```python
from build123d import *

# Parameters (mm, degrees)
F0_R     = 1.397
F1_DEPTH = 3.048


with BuildPart() as f1:
    # F0 (on Front) → F1 (new body)
    with BuildSketch(Plane.XZ):
        with BuildLine():
            ThreePointArc((3.175, 66.675), (-2.245064, 68.920064), (0, 63.5))
            ThreePointArc((0, 63.5), (2.245064, 64.429936), (3.175, 66.675))
        make_face()
        with BuildLine():
            ThreePointArc((0, 57.15), (6.735192, 59.939808), (9.525, 66.675))
            ThreePointArc((9.525, 66.675), (0.596483, 76.181305), (-9.450293, 67.865625))
            ThreePointArc((-9.450293, 67.865625), (-7.14375, 60.374805), (0, 57.15))
        make_face()
        with BuildLine():
            ThreePointArc((3.175, 66.675), (2.245064, 64.429936), (0, 63.5))
            ThreePointArc((0, 63.5), (-2.245064, 68.920064), (3.175, 66.675))
        make_face(mode=Mode.SUBTRACT)
        with BuildLine():
            Line((15.747457, 17.883289), (9.525, 66.675))
            ThreePointArc((9.525, 66.675), (6.735192, 59.939808), (0, 57.15))
            Line((0, 57.15), (0, 31.75))
            ThreePointArc((0, 31.75), (10.491283, 27.789219), (15.747457, 17.883289))
        make_face()
        with BuildLine():
            ThreePointArc((0, 57.15), (-7.14375, 60.374805), (-9.450293, 67.865625))
            Line((-9.450293, 67.865625), (-15.750488, 17.859375))
            ThreePointArc((-15.750488, 17.859375), (-10.500326, 27.78125), (0, 31.75))
            Line((0, 31.75), (0, 57.15))
        make_face()
        with Locations((-3.175, 52.4002)):
            Circle(F0_R, mode=Mode.SUBTRACT)
        with BuildLine():
            ThreePointArc((15.875, 15.875), (15.843082, 16.881168), (15.747457, 17.883289))
            ThreePointArc((15.747457, 17.883289), (10.491283, 27.789219), (0, 31.75))
            Line((0, 31.75), (0, 17.653))
            ThreePointArc((0, 17.653), (1.257236, 17.132236), (1.778, 15.875))
            ThreePointArc((1.778, 15.875), (1.257236, 14.617764), (0, 14.097))
            Line((0, 14.097), (0, 0))
            ThreePointArc((0, 0), (10.572083, 4.03242), (15.77332, 14.081125))
            ThreePointArc((15.77332, 14.081125), (15.84956, 14.976623), (15.875, 15.875))
        make_face()
        with BuildLine():
            ThreePointArc((0, 31.75), (-10.500326, 27.78125), (-15.750488, 17.859375))
            ThreePointArc((-15.750488, 17.859375), (-15.875, 15.875), (-15.750488, 13.890625))
            ThreePointArc((-15.750488, 13.890625), (-10.500326, 3.96875), (0, 0))
            Line((0, 0), (0, 14.097))
            ThreePointArc((0, 14.097), (-1.778, 15.875), (0, 17.653))
            Line((0, 17.653), (0, 31.75))
        make_face()
        with BuildLine():
            ThreePointArc((0, 0), (-10.500326, 3.96875), (-15.750488, 13.890625))
            Line((-15.750488, 13.890625), (-8.643798, -48.607884))
            ThreePointArc((-8.643798, -48.607884), (-6.48968, -41.831439), (0, -38.9255))
            Line((0, -38.9255), (0, 0))
        make_face()
        with BuildLine():
            Line((10.715191, -30.394381), (15.77332, 14.081125))
            ThreePointArc((15.77332, 14.081125), (10.572083, 4.03242), (0, 0))
            Line((0, 0), (0, -38.9255))
            ThreePointArc((0, -38.9255), (0.148885, -38.926774), (0.297726, -38.930596))
            ThreePointArc((0.297726, -38.930596), (6.255852, -41.579703), (8.6995, -47.625))
            Line((8.6995, -47.625), (36.5125, -47.625))
            ThreePointArc((36.5125, -47.625), (38.885575, -41.964516), (44.585844, -39.688663))
            Line((44.585844, -39.688663), (18.478408, -39.241789))
            ThreePointArc((18.478408, -39.241789), (12.638616, -36.536307), (10.715191, -30.394381))
        make_face()
        with BuildLine():
            ThreePointArc((0, -38.9255), (-6.48968, -41.831439), (-8.643798, -48.607884))
            ThreePointArc((-8.643798, -48.607884), (-5.793561, -54.11468), (0, -56.3245))
            Line((0, -56.3245), (0.297726, -56.319404))
            ThreePointArc((0.297726, -56.319404), (6.255852, -53.670297), (8.6995, -47.625))
            Line((8.6995, -47.625), (2.032, -47.625))
            ThreePointArc((2.032, -47.625), (-1.436841, -49.061841), (0, -45.593))
            Line((0, -45.593), (0, -38.9255))
        make_face()
        with BuildLine():
            Line((0.297726, -56.319404), (0, -56.3245))
            ThreePointArc((0, -56.3245), (0.148885, -56.323226), (0.297726, -56.319404))
        make_face()
        with BuildLine():
            ThreePointArc((8.6995, -47.625), (6.255852, -53.670297), (0.297726, -56.319404))
            Line((0.297726, -56.319404), (44.585844, -55.561337))
            ThreePointArc((44.585844, -55.561337), (38.885575, -53.285484), (36.5125, -47.625))
            Line((36.5125, -47.625), (8.6995, -47.625))
        make_face()
        with BuildLine():
            ThreePointArc((46.482, -47.625), (44.45, -45.593), (42.418, -47.625))
            ThreePointArc((42.418, -47.625), (44.45, -49.657), (46.482, -47.625))
        make_face()
        with BuildLine():
            ThreePointArc((52.3875, -47.625), (50.110484, -42.060575), (44.585844, -39.688663))
            ThreePointArc((44.585844, -39.688663), (38.885575, -41.964516), (36.5125, -47.625))
            ThreePointArc((36.5125, -47.625), (38.885575, -53.285484), (44.585844, -55.561337))
            ThreePointArc((44.585844, -55.561337), (50.110484, -53.189425), (52.3875, -47.625))
        make_face()
        with BuildLine():
            ThreePointArc((46.482, -47.625), (44.45, -49.657), (42.418, -47.625))
            ThreePointArc((42.418, -47.625), (44.45, -45.593), (46.482, -47.625))
        make_face(mode=Mode.SUBTRACT)
        with BuildLine():
            Line((0.297726, -38.930596), (0, -38.9255))
            Line((0, -38.9255), (0, -45.593))
            ThreePointArc((0, -45.593), (1.436841, -46.188159), (2.032, -47.625))
            Line((2.032, -47.625), (8.6995, -47.625))
            ThreePointArc((8.6995, -47.625), (6.255852, -41.579703), (0.297726, -38.930596))
        make_face()
    extrude(amount=F1_DEPTH)


solid = f1.part
```
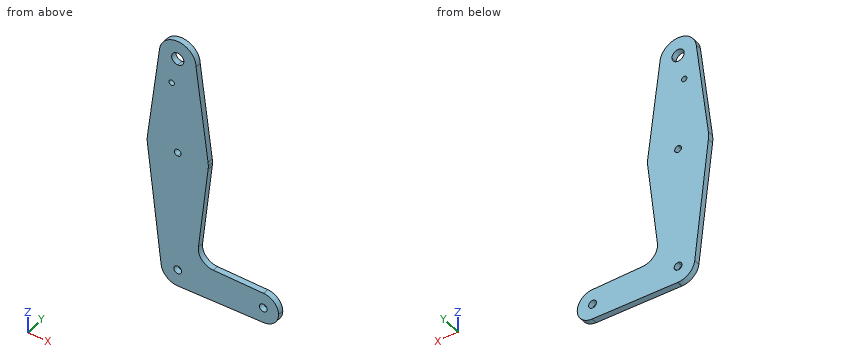
Check sheet for the modelled part. Datum: model origin and axes. Units: mm. Give positions to 0.01 mm unless a question says otherwise; leave off trailing zeros. Loops run counter-clockwise (first coordinate to the right, second up) from the corner with the lowest first, then second, coordinate; pieces in that order, holes last. Notation, with made-up numbers: (83.25, 65) - (89.25, 65) arc R28 cw to (89.25, 91) - close; hole circle Ø4 at (-28.5, 74.5). An arc over 180 degrees is marked (long way). One line per question, with ' | ' between items. Start each with the question number.
1. Cross-section at D-D, the plane x = -6. Enter the section's corners in (y, z), plus the area to 3 significant figures.
2. Cross-section at A-A, the plane x = 12. Enter the section's corners in (y, z).
3. Cross-section at C-C, the plane z = 42. Enter the section's corners in (x, y), plus the area to 3 significant figures.
4. Material ranges on line 1 along X through (y, z) = (-1.5, -49); line 2 along X through (y, z) = (-1.4, -46); line 3 along Z through (x, y) = (44.45, -2.4), recorded low to high. Write a range as [from, to].
5. Gauge pin test, flat ends, axial feed: pin 1 Ø1.5 at (y, z) = (-2, 57.5) entering from +X; pin 2 Ø1 at (x, y) = (31, -0.5) entering from +Z. Record the tip position at first contact, or that the pin passes through.
Check result:
1) outline: (-3.05, -53.92) - (0, -53.92) - (0, 74.07) - (-3.05, 74.07) - close | area: 390 mm2
2) outline: (-3.05, -56.12) - (0, -56.12) - (0, -35.7) - (-3.05, -35.7) - close; (-3.05, -19.1) - (0, -19.1) - (0, 47.27) - (-3.05, 47.27) - close
3) outline: (-12.71, -3.05) - (12.67, -3.05) - (12.67, 0) - (-12.71, 0) - close | area: 77.4 mm2
4) line 1: x = [-8.59, -1.5], [1.5, 42.95], [45.95, 52.27] | line 2: x = [-8.94, -1.22], [1.22, 43.23], [45.67, 52.22] | line 3: z = [-55.56, -49.66], [-45.59, -39.69]
5) pin 1: stops at x = 10.79 | pin 2: stops at z = -39.45
